Verification items for the finished model (mm, model axes). A direction names the side the tool comes from. Round coordinates to 2 decimals unless told otherwise and drop trailing zeros. Order: outer loops, then holes, each group sorted by start corner. A loop starts at its lowest first (then second) coordinate and runs counter-clockwise, first axis right, second up.
```python
from build123d import *

# Parameters (mm, degrees)
F1_DEPTH = 50.8


with BuildPart() as f1:
    # F0 (on Front) → F1 (new body)
    with BuildSketch(Plane.XZ):
        with BuildLine():
            Line((-46.61043, 29.230101), (-78.36043, 29.230101))
            Line((-78.36043, 29.230101), (-78.36043, 27.642601))
            ThreePointArc((-78.36043, 27.642601), (-77.895462, 26.520069), (-76.77293, 26.055101))
            Line((-76.77293, 26.055101), (-49.78543, 26.055101))
            Line((-49.78543, 26.055101), (-49.78543, -13.632399))
            ThreePointArc((-49.78543, -13.632399), (-49.320462, -14.754931), (-48.19793, -15.219899))
            Line((-48.19793, -15.219899), (-46.61043, -15.219899))
            Line((-46.61043, -15.219899), (-46.61043, 29.230101))
        make_face()
    extrude(amount=F1_DEPTH)


solid = f1.part
```
1) Sectioned sample at C-C on x = -71. Record the cut outline in (y, z), then the cut area to 3 significant figures.
2) Sectioned sample at A-A on y = -15. Record the cut outline in (x, z) (1 decimal).
3) Go/stop test with flat-tipped pins: pin 1 Ø4 at (x, y) = (-60.5, -27.5) entering from -Z; pin 2 Ø2 at (y, z) = (-24, 13) entering from -X. Record where each tip stops, or that it passes through.
4) Scan lines: probe 1 along Z at (x, y) = (-61, -31); probe 2 along X at (y, z) = (-34, 21); probe 3 along Z at (x, y) = (-48.5, -12). Record each from-to range of solid material in increasing order.
5) Sectioned sample at B-B on z = 14.5. Record the cut outline in (x, y).
6) Tool access check on faces 1 (the flat face through (-63, -25, 26.055)), 2 (the flat face through (-49.6, -50.8, 15.3)). Record the directions out of +Z, -Z, +X, -X, +Y, -Y that give a thin tool (end or side, any length) a straight path to the whole face; none if there is none.
Returned:
1. outline: (-50.8, 26.06) - (0, 26.06) - (0, 29.23) - (-50.8, 29.23) - close
1. area: 161 mm2
2. outline: (-78.4, 27.6) arc R1.6 ccw to (-76.8, 26.1) - (-49.8, 26.1) - (-49.8, -13.6) arc R1.6 ccw to (-48.2, -15.2) - (-46.6, -15.2) - (-46.6, 29.2) - (-78.4, 29.2) - close
3. pin 1: stops at z = 26.06
3. pin 2: stops at x = -49.79
4. probe 1: z = 26.06 to 29.23
4. probe 2: x = -49.79 to -46.61
4. probe 3: z = -15.19 to 29.23
5. outline: (-49.79, -50.8) - (-46.61, -50.8) - (-46.61, 0) - (-49.79, 0) - close
6. face 1: -Z, -X, +Y, -Y
6. face 2: +Z, -Z, +X, -X, -Y
